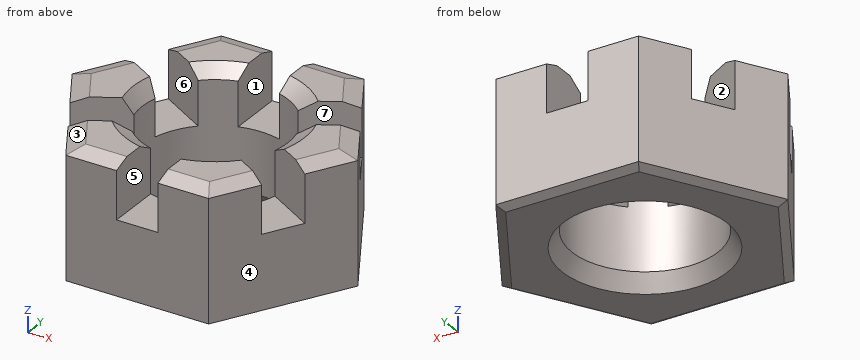
from build123d import *
from OCP.BRepFilletAPI import BRepFilletAPI_MakeChamfer

# Parameters (mm, degrees)
RESSALTO_EXTRUS_O1_DEPTH = 16
CHANFRO1_SIZE            = 2
CHANFRO1_SIZE2           = 0.727940469
ESBO_O2_R                = 8.8
CORTE_EXTRUS_O1_DEPTH    = 16
ESBO_O3_W                = 5
ESBO_O3_H                = 10
CORTE_EXTRUS_O2_DEPTH    = 6.5
CHANFRO2_SIZE            = 2
CHANFRO2_SIZE2           = 1.154700538
CHANFRO3_SIZE            = 2
CHANFRO3_SIZE2           = 1.154700538
CHANFRO5_SIZE            = 1
CHANFRO5_SIZE2           = 0.577350269


with BuildPart() as part:
    # Esboço1 → Ressalto-extrusão1 (new body)
    with BuildSketch(Plane.XY):
        Polygon((17.320508076, 0), (8.660254038, 15), (-8.660254038, 15), (-17.320508076, 0), (-8.660254038, -15), (8.660254038, -15), align=None)
    extrude(amount=RESSALTO_EXTRUS_O1_DEPTH)

    # Chanfro1
    chanfro1_edges = [part.edges().sort_by_distance(p)[0] for p in [
        (0, 15, 16),
        (-12.990381057, 7.5, 16),
        (-12.990381057, -7.5, 16),
        (0, -15, 16),
        (12.990381057, -7.5, 16),
        (12.990381057, 7.5, 16),
    ]]
    chanfro1_side = [part.faces().sort_by_distance(p)[0] for p in [
        (0, 0, 16),
    ]]
    chamfer(chanfro1_edges, length=CHANFRO1_SIZE, length2=CHANFRO1_SIZE2, reference=chanfro1_side[0])

    # Esboço2 → Corte-extrusão1 (cut)
    with BuildSketch(Plane.XY.offset(16)):
        Circle(ESBO_O2_R)
    extrude(amount=-CORTE_EXTRUS_O1_DEPTH, mode=Mode.SUBTRACT)

    # Esboço3 → Corte-extrusão2 (cut)
    with BuildSketch(Plane.XY.offset(16)):
        Polygon((13.353868008, 10.596610635), (15.853868008, 6.266483616), (7.19361397, 1.266483616), (4.69361397, 5.596610635), align=None)
        with Locations((0, 11.863094251)):
            Rectangle(ESBO_O3_W, ESBO_O3_H)
        Polygon((15.853868008, -6.266483616), (13.353868008, -10.596610635), (4.69361397, -5.596610635), (7.19361397, -1.266483616), align=None)
        with Locations((0, -11.863094251)):
            Rectangle(ESBO_O3_W, ESBO_O3_H)
        Polygon((-13.353868008, -10.596610635), (-15.853868008, -6.266483616), (-7.19361397, -1.266483616), (-4.69361397, -5.596610635), align=None)
        Polygon((-15.853868008, 6.266483616), (-13.353868008, 10.596610635), (-4.69361397, 5.596610635), (-7.19361397, 1.266483616), align=None)
    extrude(amount=-CORTE_EXTRUS_O2_DEPTH, mode=Mode.SUBTRACT)

    # Chanfro2: one chamfer whose edges measure the first distance from different faces: ONE call of the kernel's chamfer builder (chamfer() names one face for all edges)
    chanfro2_edges_1 = [part.edges().sort_by_distance(p)[0] for p in [
        (4.4, -7.621023553, 16),
    ]]
    chanfro2_side_1 = [part.faces().sort_by_distance(p)[0] for p in [
        (5.798091402, -10.042588894, 16),
    ]]
    chanfro2_edges_2 = [part.edges().sort_by_distance(p)[0] for p in [
        (-4.4, -7.621023553, 16),
    ]]
    chanfro2_side_2 = [part.faces().sort_by_distance(p)[0] for p in [
        (-5.798091402, -10.042588894, 16),
    ]]
    chanfro2_edges_3 = [part.edges().sort_by_distance(p)[0] for p in [
        (-8.8, 0, 16),
    ]]
    chanfro2_side_3 = [part.faces().sort_by_distance(p)[0] for p in [
        (-8.8, 0, 8),
    ]]
    chanfro2_edges_4 = [part.edges().sort_by_distance(p)[0] for p in [
        (-4.4, 7.621023553, 16),
    ]]
    chanfro2_side_4 = [part.faces().sort_by_distance(p)[0] for p in [
        (-5.798091402, 10.042588894, 16),
    ]]
    chanfro2_edges_5 = [part.edges().sort_by_distance(p)[0] for p in [
        (4.4, 7.621023553, 16),
    ]]
    chanfro2_side_5 = [part.faces().sort_by_distance(p)[0] for p in [
        (5.798091402, 10.042588894, 16),
    ]]
    chanfro2_edges_6 = [part.edges().sort_by_distance(p)[0] for p in [
        (8.739043173, 1.033984733, 16),
    ]]
    chanfro2_side_6 = [part.faces().sort_by_distance(p)[0] for p in [
        (11.596182803, 0, 16),
    ]]
    chanfro2 = BRepFilletAPI_MakeChamfer(part.part.solid().wrapped)
    for e in chanfro2_edges_1:
        chanfro2.Add(CHANFRO2_SIZE, CHANFRO2_SIZE2, e.wrapped, chanfro2_side_1[0].wrapped)  # the first distance lies on this face
    for e in chanfro2_edges_2:
        chanfro2.Add(CHANFRO2_SIZE, CHANFRO2_SIZE2, e.wrapped, chanfro2_side_2[0].wrapped)  # the first distance lies on this face
    for e in chanfro2_edges_3:
        chanfro2.Add(CHANFRO2_SIZE, CHANFRO2_SIZE2, e.wrapped, chanfro2_side_3[0].wrapped)  # the first distance lies on this face
    for e in chanfro2_edges_4:
        chanfro2.Add(CHANFRO2_SIZE, CHANFRO2_SIZE2, e.wrapped, chanfro2_side_4[0].wrapped)  # the first distance lies on this face
    for e in chanfro2_edges_5:
        chanfro2.Add(CHANFRO2_SIZE, CHANFRO2_SIZE2, e.wrapped, chanfro2_side_5[0].wrapped)  # the first distance lies on this face
    for e in chanfro2_edges_6:
        chanfro2.Add(CHANFRO2_SIZE, CHANFRO2_SIZE2, e.wrapped, chanfro2_side_6[0].wrapped)  # the first distance lies on this face
    add(Compound.cast(chanfro2.Shape()), mode=Mode.REPLACE)

    # Chanfro3
    chanfro3_edges = [part.edges().sort_by_distance(p)[0] for p in [
        (-8.8, 0, 0),
    ]]
    chanfro3_side = [part.faces().sort_by_distance(p)[0] for p in [
        (-8.8, 0, 7.422649731),
    ]]
    chamfer(chanfro3_edges, length=CHANFRO3_SIZE, length2=CHANFRO3_SIZE2, reference=chanfro3_side[0])

    # Chanfro5
    chanfro5_edges = [part.edges().sort_by_distance(p)[0] for p in [
        (0, -15, 0),
        (-12.990381057, -7.5, 0),
        (-12.990381057, 7.5, 0),
        (0, 15, 0),
        (12.990381057, 7.5, 0),
        (12.990381057, -7.5, 0),
    ]]
    chanfro5_side = [part.faces().sort_by_distance(p)[0] for p in [
        (-10.412958108, 0, 0),
    ]]
    chamfer(chanfro5_edges, length=CHANFRO5_SIZE, length2=CHANFRO5_SIZE2, reference=chanfro5_side[0])


solid = part.part
Design review of the part built by this model. Coordinates are the model's own, in mm. Face numbers are marked on the shaded views. A direction names the side the tool comes from. Coordinates: 2 decimals unless noted, no trailing zeros. Order: outer loops, then holes, each group sorted by start corner. A loop starts at its lowest first (then second) coordinate and runs counter-clockwise, first axis right, second up. Notation, with made-up numbers: M 88,-33 L 137,-33 A22 ccw 137,-2 Z; hole C -1,-24 d2. An arc over 180 degrees is marked long. Use a Markdown table: item, result.
(1) Add section B-B (z = 2.5). Give the boundary of the cut face in (x, y), then the cut area to 3 significant figures.
Worked answers:
| item | result |
|---|---|
| outline | M -17.32,0 L -8.66,-15 L 8.66,-15 L 17.32,0 L 8.66,15 L -8.66,15 Z; hole C 0,0 d17.6 |
| area | 536 mm2 |
(2) Add section A-A (x = 0). Give the boundary of the cut face in (y, z), then the cut area to 3 significant figures.
Worked answers:
| item | result |
|---|---|
| outline | M -15,0.58 L -14,0 L -9.95,0 L -8.8,2 L -8.8,9.5 L -15,9.5 Z; M 8.8,2 L 9.95,0 L 14,0 L 15,0.58 L 15,9.5 L 8.8,9.5 Z |
| area | 115 mm2 |
(3) Wall thickness on probe 1 along Y at (x, z) = (0, 7.5); probe 2 along Y at (x, z) = (8, 12.25); probe 3 along X at (y, z) = (-7, 8.25): over which ranges is each line inside the solid? List them lowest first.
Worked answers:
| item | result |
|---|---|
| probe 1 | y = -15 to -8.8, 8.8 to 15 |
| probe 2 | y = -15 to -7.51, 7.51 to 15 |
| probe 3 | x = -13.28 to -5.33, 5.33 to 13.28 |
(4) For P1, Ø3, axis at y = 12, z = 12.5, coming from the +X side; P2, Ø2, axis at y = -13, z = 14, coming from the -X side; P3, Ø2.5, axis at x = -10.5, y = 6, coming from the +Z side, all flat-tipped, find the tip position at first contact; note any pin that passes through.
Worked answers:
| item | result |
|---|---|
| P1 | stops at x = 11.26 |
| P2 | stops at x = -10.39 |
| P3 | stops at z = 9.5 |
(5) Draft analysis for pull direction Y (two halves, no side actions). For the marked faces 4, 5, 6 and 7, state which applies: released by +Y, released by -Y, zero draft, split by the parting line, or undercut.
Worked answers:
| item | result |
|---|---|
| face 4 | released by -Y |
| face 5 | zero draft |
| face 6 | undercut |
| face 7 | undercut |
(6) Add section C-C (x = -11). Give the boundary of the cut face in (y, z), then the cut area to 3 significant figures.
Worked answers:
| item | result |
|---|---|
| outline | M -10.95,0.58 L -8.95,0 L 8.95,0 L 10.95,0.58 L 10.95,15.27 L 9.24,15.58 L 9.24,9.5 L 3.46,9.5 L 3.46,16 L -3.46,16 L -3.46,9.5 L -9.24,9.5 L -9.24,15.58 L -10.95,15.27 Z |
| area | 272 mm2 |
(7) For the marked faces 1, 2 and 3, list the 3-axis set-ups (+Z, -Z, +X, -X, +Y, -Y) from which the entire face can be reached by the end or side of a thin tool; tool diameter is ignored.
Worked answers:
| item | result |
|---|---|
| face 1 | +Z, +Y, -Y |
| face 2 | +Z |
| face 3 | +Z, -X, -Y |
